from build123d import *

# Parameters (mm, degrees)
SKETCH1_W           = 120
SKETCH1_H           = 140
BOSS_EXTRUDE1_DEPTH = 3
SKETCH2_R           = 1.5
CUT_EXTRUDE1_DEPTH  = 107.343782141
SKETCH3_R           = 1.5
CUT_EXTRUDE3_DEPTH  = 107.343782141
SKETCH4_R           = 1.5
CUT_EXTRUDE4_DEPTH  = 107.343782141
SKETCH5_R           = 1.5
CUT_EXTRUDE5_DEPTH  = 3
SKETCH6_R           = 1.525
SKETCH6_W           = 10
SKETCH6_H           = 2.05
SKETCH6_W_2         = 20
CUT_EXTRUDE7_DEPTH  = 107.343782141
SKETCH9_R           = 1.525
CUT_EXTRUDE8_DEPTH  = 3
SKETCH10_W          = 44
SKETCH10_H          = 12
CUT_EXTRUDE9_DEPTH  = 5
SKETCH11_R          = 1.5
CUT_EXTRUDE10_DEPTH = 5
SKETCH12_W          = 2.05
SKETCH12_H          = 20
CUT_EXTRUDE11_DEPTH = 10


with BuildPart() as part:
    # Sketch1 → Boss-Extrude1 (new body)
    with BuildSketch(Plane(origin=(0, 0, 0), x_dir=(1, 0, 0), z_dir=(0, 1, 0))):
        Rectangle(SKETCH1_W, SKETCH1_H)
        Polygon((-80, 21.791828604), (-60, 10), (-60, 70), (-80, 70), align=None)
        Polygon((80, 70), (60, 70), (60, 10), (80, 21.791828604), align=None)
    extrude(amount=BOSS_EXTRUDE1_DEPTH)

    # Sketch2 → Cut-Extrude1 (cut, through all)
    with BuildSketch(Plane(origin=(0, 3, 0), x_dir=(1, 0, 0), z_dir=(0, 1, 0))):
        with Locations(Location((-38, -60, 0), (0, 0, 270))):
            Circle(SKETCH2_R)
        with Locations(Location((-25, -27, 0), (0, 0, 270))):
            Circle(SKETCH2_R)
        with Locations(Location((5, -27, 0), (0, 0, 270))):
            Circle(SKETCH2_R)
        with Locations(Location((-8, -60, 0), (0, 0, 270))):
            Circle(SKETCH2_R)
        with Locations(Location((35, -27, 0), (0, 0, 270))):
            Circle(SKETCH2_R)
        with Locations(Location((22, -60, 0), (0, 0, 270))):
            Circle(SKETCH2_R)
    extrude(amount=-CUT_EXTRUDE1_DEPTH, mode=Mode.SUBTRACT)

    # Sketch3 → Cut-Extrude3 (cut, through all)
    with BuildSketch(Plane(origin=(0, 3, 0), x_dir=(1, 0, 0), z_dir=(0, 1, 0))):
        with Locations(Location((-27.529579069, 60.385555627, 0), (0, 0, 270))):
            Circle(SKETCH3_R)
        with Locations(Location((-27.529579069, 7.385555627, 0), (0, 0, 90))):
            Circle(SKETCH3_R)
        with Locations(Location((27.470420931, 7.385555627, 0), (0, 0, 270))):
            Circle(SKETCH3_R)
        with Locations(Location((27.470420931, 60.385555627, 0), (0, 0, 90))):
            Circle(SKETCH3_R)
    extrude(amount=-CUT_EXTRUDE3_DEPTH, mode=Mode.SUBTRACT)

    # Sketch4 → Cut-Extrude4 (cut, through all)
    with BuildSketch(Plane(origin=(0, 3, 0), x_dir=(1, 0, 0), z_dir=(0, 1, 0))):
        with Locations(Location((-75, 34.863883517, 0), (0, 0, 270))):
            Circle(SKETCH4_R)
        with Locations(Location((-75, 58.863883517, 0), (0, 0, 270))):
            Circle(SKETCH4_R)
        with Locations(Location((-46, 34.863883517, 0), (0, 0, 90))):
            Circle(SKETCH4_R)
        with Locations(Location((-46, 58.863883517, 0), (0, 0, 90))):
            Circle(SKETCH4_R)
        with Locations(Location((46, 58.863883517, 0), (0, 0, 270))):
            Circle(SKETCH4_R)
        with Locations(Location((46, 34.863883517, 0), (0, 0, 270))):
            Circle(SKETCH4_R)
        with Locations(Location((75, 34.863883517, 0), (0, 0, 90))):
            Circle(SKETCH4_R)
        with Locations(Location((75, 58.863883517, 0), (0, 0, 90))):
            Circle(SKETCH4_R)
    extrude(amount=-CUT_EXTRUDE4_DEPTH, mode=Mode.SUBTRACT)

    # Sketch5 → Cut-Extrude5 (cut)
    with BuildSketch(Plane(origin=(0, 3, 0), x_dir=(1, 0, 0), z_dir=(0, 1, 0))):
        with Locations(Location((-68, 30, 0), (0, 0, 270))):
            Circle(SKETCH5_R)
        with Locations(Location((-53, 30, 0), (0, 0, 270))):
            Circle(SKETCH5_R)
    extrude(amount=-CUT_EXTRUDE5_DEPTH, mode=Mode.SUBTRACT)

    # Sketch6 → Cut-Extrude7 (cut, through all)
    with BuildSketch(Plane(origin=(0, 3, 0), x_dir=(1, 0, 0), z_dir=(0, 1, 0))):
        with Locations(Location((-53, -64.8, 0), (0, 0, 270))):
            Circle(SKETCH6_R)
        with Locations(Location((53, -64.8, 0), (0, 0, 90))):
            Circle(SKETCH6_R)
        with Locations((-40, -53.975)):
            Rectangle(SKETCH6_W, SKETCH6_H)
        with Locations((40, -53.975)):
            Rectangle(SKETCH6_W, SKETCH6_H)
        with Locations((30, -21.725)):
            Rectangle(SKETCH6_W_2, SKETCH6_H)
        with Locations((-30, -21.725)):
            Rectangle(SKETCH6_W_2, SKETCH6_H)
        with Locations((35, 23.325)):
            Rectangle(SKETCH6_W, SKETCH6_H)
        with Locations((-35, 23.325)):
            Rectangle(SKETCH6_W, SKETCH6_H)
    extrude(amount=-CUT_EXTRUDE7_DEPTH, mode=Mode.SUBTRACT)

    # Sketch9 → Cut-Extrude8 (cut)
    with BuildSketch(Plane(origin=(0, 3, 0), x_dir=(1, 0, 0), z_dir=(0, 1, 0))):
        with Locations(Location((-54, 22, 0), (0, 0, 270))):
            Circle(SKETCH9_R)
        with Locations(Location((54, 22, 0), (0, 0, 90))):
            Circle(SKETCH9_R)
    extrude(amount=-CUT_EXTRUDE8_DEPTH, mode=Mode.SUBTRACT)

    # Sketch10 → Cut-Extrude9 (cut)
    with BuildSketch(Plane(origin=(0, 3, 0), x_dir=(1, 0, 0), z_dir=(0, 1, 0))):
        with Locations((0.046472237, -6.975074484)):
            Rectangle(SKETCH10_W, SKETCH10_H)
    extrude(amount=-CUT_EXTRUDE9_DEPTH, mode=Mode.SUBTRACT)

    # Sketch11 → Cut-Extrude10 (cut)
    with BuildSketch(Plane(origin=(0, 3, 0), x_dir=(1, 0, 0), z_dir=(0, 1, 0))):
        with Locations(Location((-53, 64, 0), (0, 0, 270))):
            Circle(SKETCH11_R)
        with Locations(Location((53, 64, 0), (0, 0, 270))):
            Circle(SKETCH11_R)
    extrude(amount=-CUT_EXTRUDE10_DEPTH, mode=Mode.SUBTRACT)

    # Sketch12 → Cut-Extrude11 (cut)
    with BuildSketch(Plane(origin=(0, 3, 0), x_dir=(1, 0, 0), z_dir=(0, 1, 0))):
        with Locations((-53.975, 5)):
            Rectangle(SKETCH12_W, SKETCH12_H)
        with Locations((-53.975, -45)):
            Rectangle(SKETCH12_W, SKETCH12_H)
        with Locations((53.975, -45)):
            Rectangle(SKETCH12_W, SKETCH12_H)
        with Locations((53.975, 5)):
            Rectangle(SKETCH12_W, SKETCH12_H)
    extrude(amount=-CUT_EXTRUDE11_DEPTH, mode=Mode.SUBTRACT)


solid = part.part
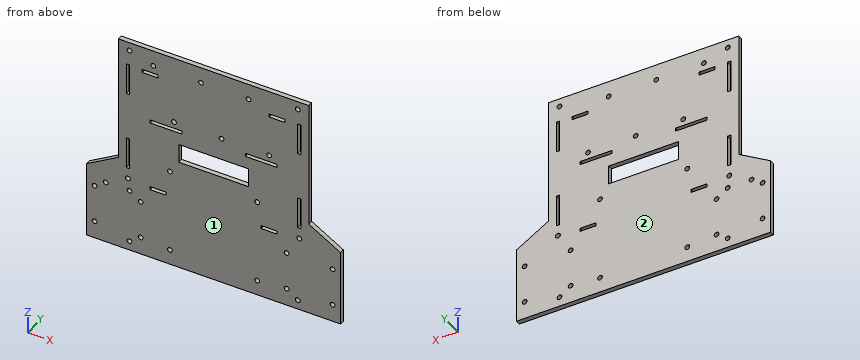
Build history of the part. All positions in model axes, mm. Face numbers are marked on the shaded views. Round coordinates to 2 decimals unless told otherwise and drop trailing zeros. Loops run counter-clockwise (first coordinate to the right, second up) from the corner with the lowest first, then second, coordinate; pieces in that order, holes last. Notation, with made-up numbers: (53, -14) -> (100, -14) arc R18 ccw to (100, -8) -> close; hole circle Ø1 at (77.5, -4.5). An arc over 180 degrees is marked (long way). One line per item, written item: value. Start each with the question number.
Q1. Probe line 1 along X through (y, z) = (0.9, 60); line 2 along X through (y, z) = (2.5, 22); line 3 along X through (y, z) = (1.25, -22) (3 decimals). List the from-to ranges inside material, lowest first.
Q2. Cut at C-C on z = 31.5. List the corners of the cut face in (x, y).
Q3. Cut at D-D on x = 68.5. List the corners of the cut face in (y, z).
Q4. Drop flat-ended pins along their axis: pin 1 Ø1 at (y, z) = (1.5, 54) entering from +X; pin 2 Ø12 at (x, z) = (-15.5, 52.5) entering from -Y; pin 3 Ø0.6 at (y, z) = (2, 22) entering from -X; pin 4 Ø2.5 at (x, z) = (-75, -58.86) entering from -Y. Give the stop position or say it passes through.
Q5. Cut at B-B on y = 0.5. Count the separate pieces of the cut face and the enclosed holes in it, plus the area to 3 significant figures.
Q6. Cut at A-A on z = -2.5. List the corners of the cut face in (x, y).
Q7. Two-plate mould, pull along Y, no slides. Class the marked faces 1 and 2: released by +Y, released by -Y, zero draft, split by the parting line, or undercut.
Computed:
1. line 1: -60 to -39.5, -36.5 to -9.5, -6.5 to 20.5, 23.5 to 60
1. line 2: -60 to -40, -20 to 20, 40 to 60
1. line 3: -80 to -55.525, -52.475 to 52.475, 55.525 to 80
2. outline: (-60, 0) -> (60, 0) -> (60, 3) -> (-60, 3) -> close
3. outline: (0, -70) -> (3, -70) -> (3, -15.01) -> (0, -15.01) -> close
4. pin 1: x = 60
4. pin 2: y = 0
4. pin 3: x = -60
4. pin 4: through
5. separate pieces: 1
5. enclosed holes: 37
5. area: 17,900 mm²
6. outline: (-60, 0) -> (-55, 0) -> (-55, 3) -> (-60, 3) -> close; (-52.95, 0) -> (52.95, 0) -> (52.95, 3) -> (-52.95, 3) -> close; (55, 0) -> (60, 0) -> (60, 3) -> (55, 3) -> close
7. face 1: released by -Y
7. face 2: released by +Y
